from build123d import *

# Parameters (mm, degrees)
SKETCH_1_W         = 10
SKETCH_1_H         = 10
EXTRUDE_1_DEPTH    = 5
HOLE_WIZARD_M3_1_D = 2.5
HOLE_WIZARD_M3_2_D = 2.5
HOLE_WIZARD_M3_3_D = 2.5
FILLET_1_R         = 1
CHAMFER_1_SIZE     = 0.2


with BuildPart() as part:
    # 草图1 → 凸台-拉伸1 (new body, symmetric)
    with BuildSketch(Plane(origin=(0, 0, 0), x_dir=(1, 0, 0), z_dir=(0, 1, 0))):
        Rectangle(SKETCH_1_W, SKETCH_1_H)
    extrude(amount=EXTRUDE_1_DEPTH, both=True)

    # M3 螺纹孔1 (through all)
    with Locations(Plane(origin=(0, 5, 0), x_dir=(1, 0, 0), z_dir=(0, 1, 0))):
        with Locations((0, 0)):
            Hole(HOLE_WIZARD_M3_1_D / 2)

    # M3 螺纹孔2 (through all)
    with Locations(Plane.XY.offset(5)):
        with Locations((0, 0)):
            Hole(HOLE_WIZARD_M3_2_D / 2)

    # M3 螺纹孔3 (through all)
    with Locations(Plane(origin=(5, 0, 0), x_dir=(0, 0, -1), z_dir=(1, 0, 0))):
        with Locations((0, 0)):
            Hole(HOLE_WIZARD_M3_3_D / 2)

    # 圆角1
    fillet_1_edges = [part.edges().sort_by_distance(p)[0] for p in [
        (5, 0, 5),
        (-5, 0, 5),
        (-5, 0, -5),
        (5, 0, -5),
    ]]
    fillet(fillet_1_edges, radius=FILLET_1_R)

    # 倒角1
    chamfer_1_edges = [part.edges().sort_by_distance(p)[0] for p in [
        (0, -5, -5),
        (0, 5, -5),
        (5, -5, 0),
        (0, -5, 5),
        (-5, -5, 0),
        (-4.707106781, -5, -4.707106781),
        (-4.707106781, -5, 4.707106781),
        (4.707106781, -5, 4.707106781),
        (4.707106781, -5, -4.707106781),
        (5, 5, 0),
        (-5, 5, 0),
        (0, 5, 5),
        (-4.707106781, 5, -4.707106781),
        (-4.707106781, 5, 4.707106781),
        (4.707106781, 5, 4.707106781),
        (4.707106781, 5, -4.707106781),
    ]]
    chamfer(chamfer_1_edges, length=CHAMFER_1_SIZE)


solid = part.part
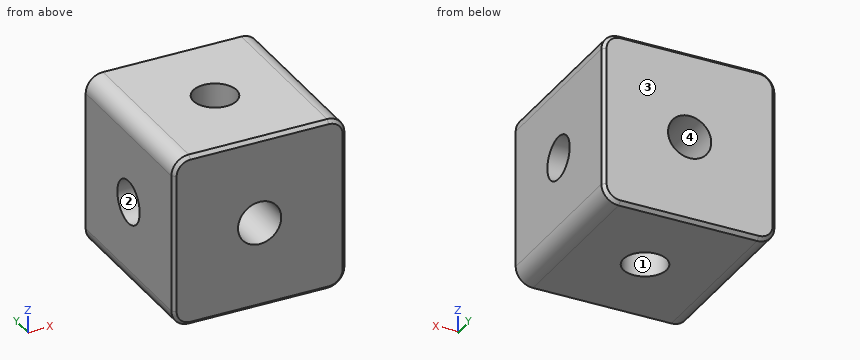
The listing builds one solid part. Answer for the finished solid, in the listing's coordinates (mm). Face numbers are marked on the shaded views. Coordinates: 2 decimals unless noted, no trailing zeros. Write each loop counter-clockwise with the first axis right and the second up, starting at its lowest first coordinate (ties: lowest second). Pieces come first, ordered by that corner, then holes. Notation, with made-up numbers: (6, 61.5) - (63, 61.5) arc R32 ccw to (63, 88.5) - close; hole circle Ø7 at (36, -14.75). An arc over 180 degrees is marked (long way). Return JSON: item names as keys, results as strings.
1. The part is cut by section B-B on y = 0. Determine the outline of the cut face in (x, z), then the cut area to 3 significant figures.
Final values:
{"outline": "(-5, -4) arc R1 ccw to (-4, -5) - (-1.25, -5) - (-1.25, -1.25) - (-5, -1.25) - close; (-5, 1.25) - (-1.25, 1.25) - (-1.25, 5) - (-4, 5) arc R1 ccw to (-5, 4) - close; (1.25, -5) - (4, -5) arc R1 ccw to (5, -4) - (5, -1.25) - (1.25, -1.25) - close; (1.25, 1.25) - (5, 1.25) - (5, 4) arc R1 ccw to (4, 5) - (1.25, 5) - close", "area": "55.4 mm^2"}
2. The part is cut by section D-D on y = 2.75. Determine the outline of the cut face in (x, z), then the cut area to 3 significant figures.
Final values:
{"outline": "(-5, -4) arc R1 ccw to (-4, -5) - (4, -5) arc R1 ccw to (5, -4) - (5, 4) arc R1 ccw to (4, 5) - (-4, 5) arc R1 ccw to (-5, 4) - close; hole circle Ø2.5 at (0, 0)", "area": "94.2 mm^2"}
3. This flat-tipped pin is pushed along its axis until it touches: pin 1 Ø3 at (x, z) = (0, 0) entering from +Y. Where does it stop, or does it pass through?
Final values:
{"pin 1": "y = 5"}
4. The part is cut by section C-C on x = -3.75. Determine the outline of the cut face in (y, z), then the cut area to 3 significant figures.
Final values:
{"outline": "(-5, -4.8) - (-4.8, -5) - (4.8, -5) - (5, -4.8) - (5, 4.8) - (4.8, 5) - (-4.8, 5) - (-5, 4.8) - close; hole circle Ø2.5 at (0, 0)", "area": "95.0 mm^2"}
5. For a pull along Y with two mould halves and no side action, classify the marked faces 1, 2, 3 and 4 as +Y half, -Y half, draft (parallel to the pull), parting line (faces both ways), or undercut.
Final values:
{"face 1": "undercut", "face 2": "undercut", "face 3": "+Y half", "face 4": "draft"}
6. Consider line 1 along Y through (x, z) = (0, 2.8); line 2 along Y through (x, z) = (4.5, 1). Determine where each line is inside the solid, lowest interval first.
Final values:
{"line 1": "-5 to -1.25, 1.25 to 5", "line 2": "-5 to -0.75, 0.75 to 5"}
7. The part is cut by section A-A on z = 0. Determine the outline of the cut face in (x, y), then the cut area to 3 significant figures.
Final values:
{"outline": "(-5, -4.8) - (-4.8, -5) - (-1.25, -5) - (-1.25, -1.25) - (-5, -1.25) - close; (-5, 1.25) - (-1.25, 1.25) - (-1.25, 5) - (-4.8, 5) - (-5, 4.8) - close; (1.25, -5) - (4.8, -5) - (5, -4.8) - (5, -1.25) - (1.25, -1.25) - close; (1.25, 1.25) - (5, 1.25) - (5, 4.8) - (4.8, 5) - (1.25, 5) - close", "area": "56.2 mm^2"}
